from build123d import *

# Parameters (mm, degrees)
SKETCH1_W               = 150
SKETCH1_H               = 120
BOSS_EXTRUDE1_DEPTH     = 15
SHELL1_T                = -2
CUT_EXTRUDE1_REACH      = 99.211
SKETCH2_W               = 120
SKETCH2_H               = 90
BOSS_EXTRUDE2_START     = -58
BOSS_EXTRUDE2_DEPTH     = 118
SKETCH4_W               = 13
SKETCH4_H               = 11
BOSS_EXTRUDE3_DEPTH     = 5
SKETCH5_R               = 2.05
CUT_EXTRUDE2_DEPTH      = 1.1
SKETCH6_W               = 10
SKETCH6_H               = 10
CUT_EXTRUDE3_DEPTH      = 2
MIRROR3_COPY_1_SKETCH_W = 13
MIRROR3_COPY_1_SKETCH_H = 11
MIRROR3_COPY_1_DEPTH    = 5
MIRROR3_COPY_2_SKETCH_R = 2.05
MIRROR3_COPY_2_DEPTH    = 1.1
FILLET1_R               = 5


with BuildPart() as part:
    # Sketch1 → Boss-Extrude1 (new body)
    with BuildSketch(Plane(origin=(0, 0, 0), x_dir=(0, 0, -1), z_dir=(1, 0, 0))):
        Rectangle(SKETCH1_W, SKETCH1_H)
    extrude(amount=-BOSS_EXTRUDE1_DEPTH)

    # Shell1
    shell1_openings = [part.faces().sort_by_distance(p)[0] for p in [
        (-7.5, 60, 0),
    ]]
    offset(amount=SHELL1_T, openings=shell1_openings, kind=Kind.INTERSECTION)

    # Sketch2 → Cut-Extrude1 (cut, up to next)
    with BuildSketch(Plane(origin=(0, 0, 0), x_dir=(0, 0, -1), z_dir=(1, 0, 0)), mode=Mode.PRIVATE) as cut_extrude1_sk1:
        Rectangle(SKETCH2_W, SKETCH2_H)
    cut_extrude1_tool1 = extrude(cut_extrude1_sk1.sketch, amount=-CUT_EXTRUDE1_REACH, mode=Mode.PRIVATE) & part.part
    add(cut_extrude1_tool1.solids().sort_by_distance((0, 0, 0))[0], mode=Mode.SUBTRACT)

    # Sketch3 → Boss-Extrude2 (add)
    with BuildSketch(Plane(origin=(0, 0, 0), x_dir=(1, 0, 0), z_dir=(0, 1, 0)).offset(BOSS_EXTRUDE2_START)):
        Polygon((-3.5, 63), (-2, 63), (-2, 64), (-4.5, 64), (-4.5, 61), (-3.5, 61), align=None)
    boss_extrude2 = extrude(amount=BOSS_EXTRUDE2_DEPTH)

    # Mirror1: Boss-Extrude2 across plane
    add(boss_extrude2.mirror(Plane.XY))

    # Sketch4 → Boss-Extrude3 (add)
    with BuildSketch(Plane(origin=(0, 60, 0), x_dir=(1, 0, 0), z_dir=(0, 1, 0))):
        with Locations((-8.5, 69.5)):
            Rectangle(SKETCH4_W, SKETCH4_H)
    boss_extrude3 = extrude(amount=-BOSS_EXTRUDE3_DEPTH)

    # Sketch5 → Cut-Extrude2 (cut)
    with BuildSketch(Plane(origin=(0, 60, 0), x_dir=(1, 0, 0), z_dir=(0, 1, 0))):
        with Locations(Location((-10.25, 70.75, 0), (0, 0, 270))):
            Circle(SKETCH5_R)
        with Locations(Location((-10.25, 66.25, 0), (0, 0, 270))):
            Circle(SKETCH5_R)
        with Locations(Location((-4.75, 70.75, 0), (0, 0, 270))):
            Circle(SKETCH5_R)
        with Locations(Location((-4.75, 66.25, 0), (0, 0, 270))):
            Circle(SKETCH5_R)
    cut_extrude2 = extrude(amount=-CUT_EXTRUDE2_DEPTH, mode=Mode.SUBTRACT)

    # Mirror2: Boss-Extrude3, Cut-Extrude2 across plane
    add(boss_extrude3.mirror(Plane.XY))
    add(cut_extrude2.mirror(Plane.XY), mode=Mode.SUBTRACT)

    # Sketch6 → Cut-Extrude3 (cut)
    with BuildSketch(Plane.ZY.offset(15)):
        with Locations((0, -53)):
            Rectangle(SKETCH6_W, SKETCH6_H)
    extrude(amount=-CUT_EXTRUDE3_DEPTH, mode=Mode.SUBTRACT)

    # Mirror3: Boss-Extrude3, Cut-Extrude2 across plane
    add(boss_extrude3.mirror(Plane.ZX))
    add(cut_extrude2.mirror(Plane.ZX), mode=Mode.SUBTRACT)

    # Mirror3 copy 1 sketch → Mirror3 copy 1 (add)
    with BuildSketch(Plane.XZ.offset(60)):
        with Locations((-8.5, 69.5)):
            Rectangle(MIRROR3_COPY_1_SKETCH_W, MIRROR3_COPY_1_SKETCH_H)
    extrude(amount=-MIRROR3_COPY_1_DEPTH)

    # Mirror3 copy 2 sketch → Mirror3 copy 2 (cut)
    with BuildSketch(Plane.XZ.offset(60)):
        with Locations(Location((-10.25, 70.75, 0), (0, 0, 270))):
            Circle(MIRROR3_COPY_2_SKETCH_R)
        with Locations(Location((-10.25, 66.25, 0), (0, 0, 270))):
            Circle(MIRROR3_COPY_2_SKETCH_R)
        with Locations(Location((-4.75, 70.75, 0), (0, 0, 270))):
            Circle(MIRROR3_COPY_2_SKETCH_R)
        with Locations(Location((-4.75, 66.25, 0), (0, 0, 270))):
            Circle(MIRROR3_COPY_2_SKETCH_R)
    extrude(amount=-MIRROR3_COPY_2_DEPTH, mode=Mode.SUBTRACT)

    # Fillet1
    fillet1_edges = [part.edges().sort_by_distance(p)[0] for p in [
        (-15, 0, 75),
        (-15, 0, -75),
        (0, 0, 75),
        (0, 0, -75),
    ]]
    fillet(fillet1_edges, radius=FILLET1_R)


solid = part.part
Input: part model. Units: mm. Frame: model coordinates. A direction names the side the tool comes from. Round coordinates to 2 decimals unless told otherwise and drop trailing zeros. Loops run counter-clockwise (first coordinate to the right, second up) from the corner with the lowest first, then second, coordinate; pieces in that order, holes last. Notation, with made-up numbers: M -34.5,83.25 L 13.5,83.25 A7 ccw 13.5,87.25 Z; hole C -33.5,44 d9. An arc over 180 degrees is marked long. Answer as CSV lines item,"result". Start each with the question number.
(1) Section B-B, the plane z = 19.5. Output: boundary loops of the cut face in (x, y).
(2) First-contact query: pin 1 (6.5 mm diameter, centred on x = -10.25, z = 66.25, fed in from +Y); pin 2 (1 mm diameter, centred on x = -5, z = -55, fed in from +Y); pin 3 (0.6 mm diameter, centred on x = -14, y = -55, fed in from +Z); pin 4 (1.2 mm diameter, centred on x = -5, z = 67, fed in from -Y). Flat tips, straight axial feed; report the tip coordinate or a pass-through.
(3) Section C-C, the plane y = 26. Output: boundary loops of the cut face in (x, z).
(4) Line query: line 1 (X direction, y = -59.2, z = -66.25); line 2 (Y direction, x = -1, z = 56); line 3 (X direction, y = -59.65, z = 70.75). Output: solid intervals per line, ascending. Write a range as [from, to].
(5) Draft query along Z for faces 1 (the flat face through (-7, -1, -75)), 2 (the cylindrical face through (-14, 1, 73)), 3 (the flat face through (-10, 58.9, 66)). Return one class per face: released by +Z, released by -Z, zero draft, split by the parting line, or undercut.
(6) Reachability of faces 4 (the flat face through (-15, 1, 1)), 5 (the flat face through (-5, 58.9, -66)), 6 (the cylindrical face through (-10.2, -59.5, 72.8)) from +Z, -Z, +X, -X, +Y, -Y: full face, straight path, thin tool, end or side. Return the list, or none.
(7) Section A-A, the plane z = 66.25. Output: boundary loops of the cut face in (x, y), plus the area to 3 significant figures.
Values found:
1,outline,"M -15,-60 L 0,-60 L 0,-45 L -2,-45 L -2,-58 L -13,-58 L -13,60 L -15,60 Z; M -2,45 L 0,45 L 0,60 L -2,60 Z"
2,pin 1,"stops at y = 60"
2,pin 2,"stops at y = -58"
2,pin 3,"stops at z = 73.36"
2,pin 4,"stops at y = -58.9"
3,outline,"M -15,-70 A5 ccw -10,-75 L -5,-75 A5 ccw 0,-70 L 0,-60 L -2,-60 L -2,-63 L -3.5,-63 L -3.5,-61 L -4.5,-61 L -4.5,-64 L -2,-64 L -2,-73 L -13,-73 L -13,73 L -2,73 L -2,64 L -4.5,64 L -4.5,61 L -3.5,61 L -3.5,63 L -2,63 L -2,60 L 0,60 L 0,70 A5 ccw -5,75 L -10,75 A5 ccw -15,70 Z"
4,line 1,"x = [-15, -12.3], [-8.2, -6.8], [-2.7, 0]"
4,line 2,"y = [-60, -45], [45, 60]"
4,line 3,"x = [-14.94, -12.3], [-8.2, -6.8], [-2.7, -0.06]"
5,face 1,"released by -Z"
5,face 2,"released by +Z"
5,face 3,"undercut"
6,face 4,"+Z, -Z, -X, +Y, -Y"
6,face 5,"+Y"
6,face 6,"-Y"
7,outline,"M -15,-60 L -12.3,-60 L -12.3,-58.9 L -8.2,-58.9 L -8.2,-60 L -6.8,-60 L -6.8,-58.9 L -2.7,-58.9 L -2.7,-60 L 0,-60 L 0,60 L -2.7,60 L -2.7,58.9 L -6.8,58.9 L -6.8,60 L -8.2,60 L -8.2,58.9 L -12.3,58.9 L -12.3,60 L -15,60 Z; hole M -13,-55 L -2,-55 L -2,55 L -13,55 Z"
7,area,"572 mm²"
